from build123d import *

# Parameters (mm, degrees)
SKETCH1_R           = 5
BOSS_EXTRUDE1_DEPTH = 200
CHAMFER1_SIZE       = 1
BOSS_EXTRUDE2_START = 70
SKETCH2_R           = 7
BOSS_EXTRUDE2_DEPTH = 10


with BuildPart() as part:
    # Sketch1 → Boss-Extrude1 (new body)
    with BuildSketch(Plane(origin=(0, 0, 0), x_dir=(0, 0, -1), z_dir=(1, 0, 0))):
        Circle(SKETCH1_R)
    extrude(amount=BOSS_EXTRUDE1_DEPTH)

    # Chamfer1
    chamfer1_edges = [part.edges().sort_by_distance(p)[0] for p in [
        (0, 0, 5),
    ]]
    chamfer(chamfer1_edges, length=CHAMFER1_SIZE)

    # Sketch2 → Boss-Extrude2 (add)
    with BuildSketch(Plane(origin=(0, 0, 0), x_dir=(0, 0, -1), z_dir=(1, 0, 0)).offset(BOSS_EXTRUDE2_START)):
        Circle(SKETCH2_R)
    extrude(amount=BOSS_EXTRUDE2_DEPTH)


solid = part.part
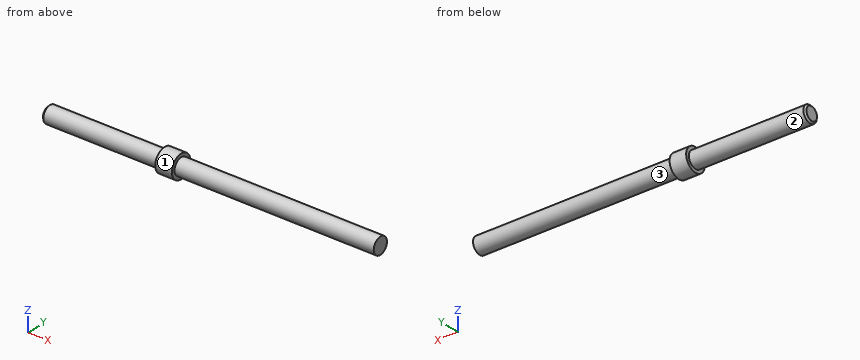
Geometry: final body of the model. Coordinates: model frame, mm. Face numbers are marked on the shaded views. A direction names the side the tool comes from. Coordinates: 2 decimals unless noted, no trailing zeros. Loops run counter-clockwise (first coordinate to the right, second up) from the corner with the lowest first, then second, coordinate; pieces in that order, holes last. Notation, with made-up numbers: (-17, 71) - (38, 71) arc R13 cw to (38, 93) - close; hole circle Ø8 at (55.25, 6). An arc over 180 degrees is marked (long way). One line per question, with ' | ' between items. Start each with the question number.
(1) First-contact query: pin 1 (5 mm diameter, centred on x = 101.5, z = 0.5, fed in from -Y); pin 2 (1 mm diameter, centred on x = 129.5, y = 3, fed in from +Z); pin 3 (4 mm diameter, centred on y = 4.5, z = 4.5, fed in from -X). Flat tips, straight axial feed; report the tip coordinate or a pass-through.
(2) Reachability of the marked faces 1, 2 and 3 from +Z, -Z, +X, -X, +Y, -Y: full face, straight path, thin tool, end or side. Return the list, or none.
(3) Ray query, L1, parallel to Y at x = 76, z = -5.75; L2, parallel to X at y = 1.25, z = 5.25; L3, parallel to Z at x = 104.5, y = -0.25. Return the intervals inside material, ascending. Write a range as from..to.
(4) Cut plane C-C on x = 46. Output: boundary loops of the cut face in (y, z).
(5) Cut plane A-A on z = 0. Output: boundary loops of the cut face in (x, y).
Here are the results:
1) pin 1: y = -5 | pin 2: z = 4.33 | pin 3: x = 0.36
2) face 1: +X, -X | face 2: -X | face 3: +X
3) L1: -3.99..3.99 | L2: 70..80 | L3: -4.99..4.99
4) outline: circle Ø10 at (0, 0)
5) outline: (0, -4) - (1, -5) - (70, -5) - (70, -7) - (80, -7) - (80, -5) - (200, -5) - (200, 5) - (80, 5) - (80, 7) - (70, 7) - (70, 5) - (1, 5) - (0, 4) - close
